Could you check a few things on this model? Use its own coordinates, in mm. Coordinates: 2 decimals unless noted, no trailing zeros. Order: outer loops, then holes, each group sorted by start corner. A loop starts at its lowest first (then second) coordinate and runs counter-clockwise, first axis right, second up. Notation, with made-up numbers: (30, 20) - (67, 20) arc R13 ccw to (67, 43) - close; hole circle Ø1 at (6, 53.5). An arc over 180 degrees is marked (long way). One line per item, written item: value.
from build123d import *

# Parameters (mm, degrees)
BOSS_EXTRUDE1_DEPTH = 10
FILLET2_R           = 30
SKETCH2_R           = 2
CUT_EXTRUDE1_DEPTH  = 10
SKETCH3_R           = 2.5
CUT_EXTRUDE2_DEPTH  = 10
SKETCH4_R           = 2.5
CUT_EXTRUDE3_DEPTH  = 11
SKETCH5_W           = 65
SKETCH5_H           = 106
CUT_EXTRUDE4_DEPTH  = 11
FILLET3_R           = 10


with BuildPart() as part:
    # Sketch1 → Boss-Extrude1 (new body)
    with BuildSketch(Plane(origin=(0, 0, 0), x_dir=(1, 0, 0), z_dir=(0, 1, 0))):
        Polygon((-47.5, 86), (-47.5, -70), (47.5, -70), (47.5, 626), (27.5, 626), (27.5, 76), (-37.5, 76), (-37.5, 86), align=None)
    extrude(amount=BOSS_EXTRUDE1_DEPTH)

    # Fillet2
    fillet2_edges = [part.edges().sort_by_distance(p)[0] for p in [
        (47.5, 5, 70),
        (-47.5, 5, 70),
    ]]
    fillet(fillet2_edges, radius=FILLET2_R)

    # Sketch2 → Cut-Extrude1 (cut)
    with BuildSketch(Plane(origin=(0, 10, 0), x_dir=(1, 0, 0), z_dir=(0, 1, 0))):
        with Locations((-42.5, 67)):
            Circle(SKETCH2_R)
        with Locations((42.5, 67)):
            Circle(SKETCH2_R)
        with Locations((7.5, -65)):
            Circle(SKETCH2_R)
    extrude(amount=-CUT_EXTRUDE1_DEPTH, mode=Mode.SUBTRACT)

    # Sketch3 → Cut-Extrude2 (cut)
    with BuildSketch(Plane(origin=(0, 10, 0), x_dir=(1, 0, 0), z_dir=(0, 1, 0))):
        with Locations((42.5, 601)):
            Circle(SKETCH3_R)
        with Locations((32.5, 611)):
            Circle(SKETCH3_R)
    extrude(amount=-CUT_EXTRUDE2_DEPTH, mode=Mode.SUBTRACT)

    # Sketch4 → Cut-Extrude3 (cut, through all)
    with BuildSketch(Plane(origin=(0, 10, 0), x_dir=(1, 0, 0), z_dir=(0, 1, 0))):
        with Locations((42.5, -25)):
            Circle(SKETCH4_R)
        with Locations((42.5, -15)):
            Circle(SKETCH4_R)
    extrude(amount=-CUT_EXTRUDE3_DEPTH, mode=Mode.SUBTRACT)

    # Sketch5 → Cut-Extrude4 (cut, through all)
    with BuildSketch(Plane(origin=(0, 10, 0), x_dir=(1, 0, 0), z_dir=(0, 1, 0))):
        with Locations((-5, 3)):
            Rectangle(SKETCH5_W, SKETCH5_H)
    extrude(amount=-CUT_EXTRUDE4_DEPTH, mode=Mode.SUBTRACT)

    # Fillet3
    fillet3_edges = [part.edges().sort_by_distance(p)[0] for p in [
        (-37.5, 5, 50),
        (27.5, 5, 50),
    ]]
    fillet(fillet3_edges, radius=FILLET3_R)


solid = part.part
Item 1: I want a section at A-A on y = 7.25. Give the number of separate pieces and of enclosed holes in the cut face, then the cut area to 3 significant figures.
Conclusion:
separate pieces: 1
enclosed holes: 8
area: 17,600 mm²
Item 2: I'm going to push flat-ended pins straight in: pin 1 Ø5 at (x, y) = (-43, 5) entering from -Z; pin 2 Ø5 at (x, z) = (7.5, 65) entering from +Y; pin 3 Ø1 at (x, y) = (23, 5) entering from +Z; pin 4 Ø3 at (y, z) = (6.5, -472) entering from -X. Where does each tip first touch, or does it pass through?
Conclusion:
pin 1: z = -86
pin 2: y = 10
pin 3: z = 69.58
pin 4: x = 27.5
Item 3: If I drill on probe 1 along X at (y, z) = (8.5, -66.5); probe 2 along Z at (x, y) = (7, 8); probe 3 along X at (y, z) = (7, 25), over which ranges is the centre line in solid material (lowest first)?
Conclusion:
probe 1: -47.5 to -44.44, -40.56 to 40.56, 44.44 to 47.5
probe 2: -76 to -56, 50 to 63.06, 66.94 to 70
probe 3: -47.5 to -37.5, 27.5 to 40, 45 to 47.5
Item 4: I want a section at B-B on z = -159.5. Please give me the cut outline in (x, y), then the cut area to 3 significant figures.
Conclusion:
outline: (27.5, 0) - (47.5, 0) - (47.5, 10) - (27.5, 10) - close
area: 200 mm²
